For this review, take the finished solid that the model builds, in its own axes (mm). Face numbers are marked on the shaded views. A direction names the side the tool comes from. Coordinates: 2 decimals unless noted, no trailing zeros. Write each loop counter-clockwise with the first axis right and the second up, starting at its lowest first coordinate (ties: lowest second). Pieces come first, ordered by that corner, then holes. Notation, with made-up numbers: (-30.5, 67) -> (23.5, 67) arc R21 cw to (23.5, 91) -> close; hole circle Ø6 at (-0.75, -19). An arc over 180 degrees is marked (long way). Put each result on its own line as item: value. Start each with the question number.
Item 1: Consider section D-D on x = 50. Give the boundary of the cut face in (y, z).
Item 2: Consider section C-C on z = -24. Give the boundary of the cut face in (x, y), and give its area (3 significant figures).
Item 3: To check wall thickness, follow L1, parallel to Z at x = 8, y = 15; L2, parallel to X at y = -0.5, z = -22.5; L3, parallel to Z at x = -49.5, y = -4. State the ranges of each line that lie inside material, in increasing order.
Item 4: Consider section B-B on y = -11. Give the boundary of the cut face in (x, z), and give its area (3 significant figures).
Item 5: Consider section A-A on x = 0. Give the boundary of the cut face in (y, z).
Item 6: Insertion check: P1, Ø9, axis at x = 2.5, y = 5.5, coming from the -Z side; P2, Ø8, axis at y = 6, z = -51, coming from the -X side; P3, Ø14, axis at x = -5, y = 9.5, coming from the -Z side; P4, Ø2, axis at y = 5.5, z = -50.5, coming from the +X side. Each pin has a flat end and moves straight along its axis. Give the tip position at first contact, or say it passes through.
Item 7: The part is to be moulded in two halves that separate along X. For the marked faces 3, 4, 5 and 6, say which applies: +X half, -X half, draft (parallel to the pull), parting line (faces both ways), or undercut.
Item 8: For the marked faces 1 and 2, list the 3-axis set-ups (+Z, -Z, +X, -X, +Y, -Y) from which the entire face can be reached by the end or side of a thin tool; tool diameter is ignored.
```python
from build123d import *

# Parameters (mm, degrees)
F0_W     = 145
F0_H     = 125
F1_DEPTH = 25
F3_R     = 17.5
F3_R_2   = 15
F4_DEPTH = 62.5
F2_W     = 30
F2_H     = 7.5
F5_DEPTH = 25
F6_DEPTH = 25
F2_R     = 18.75
F7_DEPTH = 2000
F8_DEPTH = 12500


with BuildPart() as f1:
    # F0 (on Front) → F1 (new body)
    with BuildSketch(Plane.XZ):
        Rectangle(F0_W, F0_H)
    extrude(amount=F1_DEPTH)

    # F3 (on Top) → F4 (join, symmetric)
    with BuildSketch(Plane.XY):
        Circle(F3_R)
        Circle(F3_R_2, mode=Mode.SUBTRACT)
        with Locations((50, 0)):
            Circle(F3_R)
        with Locations((50, 0)):
            Circle(F3_R_2, mode=Mode.SUBTRACT)
    extrude(amount=F4_DEPTH, both=True)

    # F2 (on face) → F5 (cut)
    with BuildSketch(Plane(origin=(0, 0, 0), x_dir=(-1, 0, 0), z_dir=(0, 1, 0))):
        with Locations((0, 50)):
            Rectangle(F2_W, F2_H)
        with Locations((0, -50)):
            Rectangle(F2_W, F2_H)
    extrude(amount=F5_DEPTH, mode=Mode.SUBTRACT)

    # F2 (on face) → F6 (cut)
    with BuildSketch(Plane(origin=(0, 0, 0), x_dir=(-1, 0, 0), z_dir=(0, 1, 0))):
        with Locations((-50, 0)):
            Rectangle(F2_W, F2_H)
    extrude(amount=F6_DEPTH, mode=Mode.SUBTRACT)

    # F2 (on face) → F7 (cut)
    with BuildSketch(Plane(origin=(0, 0, 0), x_dir=(-1, 0, 0), z_dir=(0, 1, 0))):
        with Locations((49.892824, 0)):
            Circle(F2_R)
    extrude(amount=-F7_DEPTH, mode=Mode.SUBTRACT)

    # F3 (on Top) → F8 (cut, symmetric)
    with BuildSketch(Plane.XY):
        with Locations((50, 0)):
            Circle(F3_R_2)
        Circle(F3_R_2)
    extrude(amount=F8_DEPTH, both=True, mode=Mode.SUBTRACT)


solid = f1.part
```
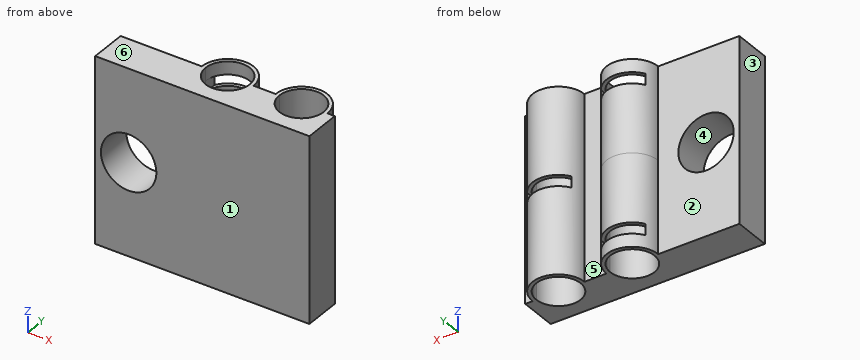
Return value:
1. outline: (-25, -62.5) -> (-15, -62.5) -> (-15, 62.5) -> (-25, 62.5) -> close; (15, -62.5) -> (17.5, -62.5) -> (17.5, -3.75) -> (15, -3.75) -> close; (15, 3.75) -> (17.5, 3.75) -> (17.5, 62.5) -> (15, 62.5) -> close
2. outline: (-72.5, -25) -> (72.5, -25) -> (72.5, 0) -> (67.5, 0) arc R17.5 ccw to (32.5, 0) -> (17.5, 0) arc R17.5 ccw to (-17.5, 0) -> (-72.5, 0) -> close; hole circle Ø30 at (0, 0); hole circle Ø30 at (50, 0)
2. area: 3,170 mm^2
3. L1: -62.5 to -53.75, -46.25 to 46.25, 53.75 to 62.5
3. L2: -72.5 to -14.99, 14.99 to 35.01, 64.99 to 72.5
3. L3: -62.5 to -18.75, 18.75 to 62.5
4. outline: (-72.5, -62.5) -> (-10.2, -62.5) -> (-10.2, 62.5) -> (-72.5, 62.5) -> close; (10.2, -62.5) -> (39.8, -62.5) -> (39.8, 62.5) -> (10.2, 62.5) -> close; (60.2, -62.5) -> (72.5, -62.5) -> (72.5, 62.5) -> (60.2, 62.5) -> close; hole circle Ø37.5 at (-49.89, 0)
4. area: 11,900 mm^2
5. outline: (-25, -62.5) -> (-15, -62.5) -> (-15, 62.5) -> (-25, 62.5) -> close; (15, -62.5) -> (17.5, -62.5) -> (17.5, -53.75) -> (15, -53.75) -> close; (15, -46.25) -> (17.5, -46.25) -> (17.5, 46.25) -> (15, 46.25) -> close; (15, 53.75) -> (17.5, 53.75) -> (17.5, 62.5) -> (15, 62.5) -> close
6. P1: through
6. P2: x = -17.39
6. P3: z = -62.5
6. P4: x = 66.91
7. face 3: -X half
7. face 4: undercut
7. face 5: undercut
7. face 6: draft
8. face 1: +Z, -Z, +X, -X, -Y
8. face 2: +Z, -Z, -X, +Y
